Verification items for this drawing (mm, ordinates from the low corner). A direction names the side the tool comes from. Give positions to 0.01 mm unless a question says otherwise; leave off trailing zeros. Loops run counter-clockwise (first coordinate to the right, second up) from the corner with the lowest first, then second, coordinate; pieces in that order, holes last. Notation, with made-up numbers: (-27, 11.5) - (-18, 11.5) arc R16 ccw to (-18, 19.5) - close; hole circle Ø3 at (84.25, -13.75). An arc over 180 degrees is marked (long way). One line per question, with ' | ' between items. Start each with the question number.
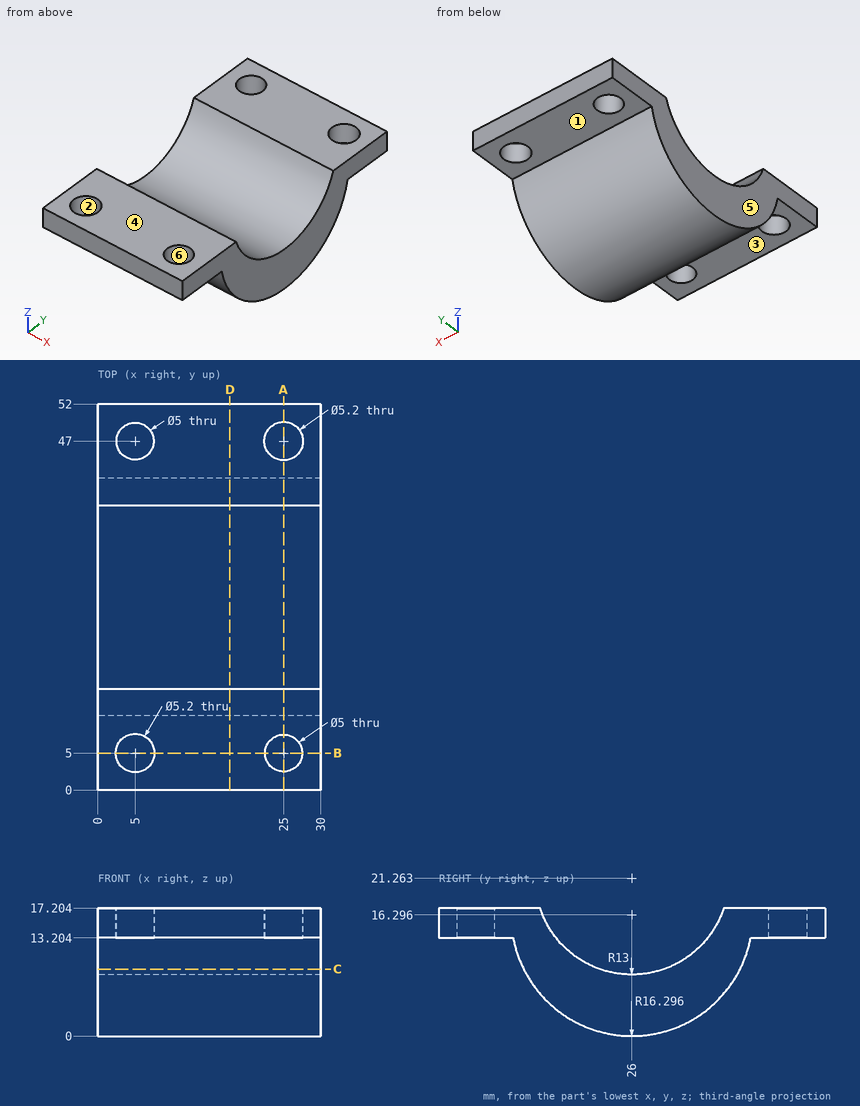
(1) Tool access check on the marked faces 1, 2 and 3. Record the directions out of +Z, -Z, +X, -X, +Y, -Y that give a thin tool (end or side, any length) a straight path to the whole face; none if there is none.
(2) Mould release check, pull along X, two halves, no side actions. Record for the marked faces 4, 5 and 6: pulls with the +X half, pulls with the -X half, needs draft (parallel to the pull), parting line crosses it, or undercut.
(3) Section check A-A, the plane x = 25. Record the boundary of the cut face in (y, z).
(4) Section check D-D, the plane x = 17.75. Record the boundary of the cut face in (y, z).
(5) Section check C-C, the plane z = 9. Record the boundary of the cut face in (x, y) (1 decimal).
(6) Material ranges on line 1 (X direction, y = 47, z = 15.55); line 2 (X direction, y = 5, z = 14.15); line 3 (Y direction, x = 25, z = 16.4) (1 decimal), recorded low to high.
(7) Section check B-B, the plane y = 5. Record the boundary of the cut face in (x, z).
(8) Depth check by flat-ended pin: pin 1 Ø6 at (x, y) = (25, 47) entering from -Z; pin 2 Ø6 at (x, y) = (12, 23.5) entering from +Z; pin 3 Ø12 at (x, y) = (20.5, 37.5) entering from -Z. Enter the tip coordinate at first touch or a pass-through.
Numbers:
1) face 1: -Z, +X, -X, +Y | face 2: +Z, -Z | face 3: -Z, +X, -X, -Y
2) face 4: needs draft | face 5: pulls with the -X half | face 6: undercut
3) outline: (0, 13.2) - (2.5, 13.2) - (2.5, 17.2) - (0, 17.2) - close; (7.5, 13.2) - (10, 13.2) arc R16.3 ccw to (42, 13.2) - (44.4, 13.2) - (44.4, 17.2) - (38.35, 17.2) arc R13 cw to (13.65, 17.2) - (7.5, 17.2) - close; (49.6, 13.2) - (52, 13.2) - (52, 17.2) - (49.6, 17.2) - close
4) outline: (0, 13.2) - (10, 13.2) arc R16.3 ccw to (42, 13.2) - (52, 13.2) - (52, 17.2) - (38.35, 17.2) arc R13 cw to (13.65, 17.2) - (0, 17.2) - close
5) outline: (0, 11.4) - (30, 11.4) - (30, 21.7) - (0, 21.7) - close; (0, 30.3) - (30, 30.3) - (30, 40.6) - (0, 40.6) - close
6) line 1: 0 to 2.5, 7.5 to 22.4, 27.6 to 30 | line 2: 0 to 2.4, 7.6 to 22.5, 27.5 to 30 | line 3: 0 to 2.5, 7.5 to 13.9, 38.1 to 44.4, 49.6 to 52
7) outline: (0, 13.2) - (2.4, 13.2) - (2.4, 17.2) - (0, 17.2) - close; (7.6, 13.2) - (22.5, 13.2) - (22.5, 17.2) - (7.6, 17.2) - close; (27.5, 13.2) - (30, 13.2) - (30, 17.2) - (27.5, 17.2) - close
8) pin 1: z = 13.2 | pin 2: z = 9.48 | pin 3: z = 0.96
